Part model, mm, in its own coordinate system. Face numbers are marked on the shaded views. A direction names the side the tool comes from. Coordinates: 2 decimals unless noted, no trailing zeros. Loops run counter-clockwise (first coordinate to the right, second up) from the corner with the lowest first, then second, coordinate; pieces in that order, holes last. Notation, with made-up numbers: M 58,1.5 L 113,1.5 A16 cw 113,11.5 Z; hole C 48,51.5 d9. An arc over 180 degrees is marked long. Answer as a JSON object with one key per item and string values. Group by question number.
1. Mould opens along Z. For the marked faces 4, 5 and 6 say: released by +Z, released by -Z, zero draft, split by the parting line, or undercut.
2. 3-axis set-ups, long thin cutter, end or side, ignore diameter. For the marked faces 1, 2 and 3: which of +Z, -Z, +X, -X, +Y, -Y reach the whole face in a straight line?
3. Saw through at D-D on z = -27.5. Write the cut outline in (x, y).
4. Saw through at A-A on z = -37.5. Write the cut outline in (x, y), then the cut area to 3 significant figures.
5. Drill centre lines: L1, parallel to Z at x = -2.25, y = 8; L2, parallel to X at y = 1.6, z = 0; L3, parallel to Y at x = 3.25, z = -36. Where is each one in solid material? Low to high.
6. Drop flat-ended pins along their axis: pin 1 Ø1 at (x, z) = (0, -4.5) entering from +Y; pin 2 Ø2.5 at (x, z) = (0, -37.5) entering from +Y; pin 3 Ø9 at (x, z) = (9.5, -12) entering from -Y; pin 4 Ø3 at (x, z) = (6.5, -2) entering from -Y. Give the stop position or say it passes through.
7. Saw through at B-B on z = -18.75. Write the cut outline in (x, y).
8. Saw through at C-C on y = 39.5. Write the cut outline in (x, z), then the cut area to 3 significant figures.
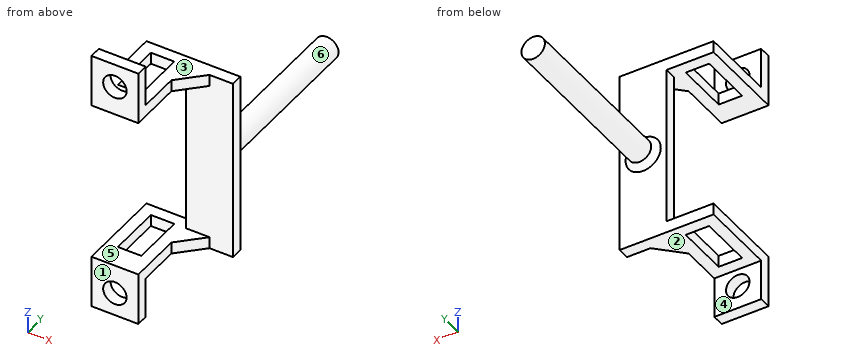
from build123d import *

# Parameters (mm, degrees)
SKETCH1_W             = 8
SKETCH1_H             = 8
SKETCH1_R             = 2
BOSS_EXTRUDE1_DEPTH   = 2
BOSS_EXTRUDE1_2_DEPTH = 2
SKETCH2_W             = 8
SKETCH2_H             = 2
BOSS_EXTRUDE2_DEPTH   = 15
BOSS_EXTRUDE3_REACH   = 43.512
SKETCH3_W             = 8
SKETCH3_H             = 2
CHAMFER1_SIZE         = 4
SKETCH4_W             = 4
SKETCH4_H             = 9
CUT_EXTRUDE1_DEPTH    = 44.026154836
SKETCH5_R             = 2
BOSS_EXTRUDE4_DEPTH   = 30
CHAMFER2_SIZE         = 1


with BuildPart() as part:
    # Sketch1 → Boss-Extrude1 (new body)
    with BuildSketch(Plane(origin=(0, 0, 0), x_dir=(1, 0, 0), z_dir=(0, 1, 0))):
        Rectangle(SKETCH1_W, SKETCH1_H)
        with Locations(Location((0, 0, 0), (0, 0, 270))):
            Circle(SKETCH1_R, mode=Mode.SUBTRACT)
    extrude(amount=BOSS_EXTRUDE1_DEPTH)



with BuildPart() as body_2:
    # Sketch1 → Boss-Extrude1 2 (new body)
    with BuildSketch(Plane(origin=(0, 0, 0), x_dir=(1, 0, 0), z_dir=(0, 1, 0))):
        with Locations((0, 37.5)):
            Rectangle(SKETCH1_W, SKETCH1_H)
        with Locations(Location((0, 37.5, 0), (0, 0, 270))):
            Circle(SKETCH1_R, mode=Mode.SUBTRACT)
    extrude(amount=BOSS_EXTRUDE1_2_DEPTH)


with BuildPart() as part_1:
    add(part.part)

    add(body_2.part)  # Boss-Extrude2 merges body 2
    # Sketch2 → Boss-Extrude2 (add)
    with BuildSketch(Plane.XZ):
        with Locations((0, -33.5)):
            Rectangle(SKETCH2_W, SKETCH2_H)
        with Locations((0, -4)):
            Rectangle(SKETCH2_W, SKETCH2_H)
    extrude(amount=-BOSS_EXTRUDE2_DEPTH)

    # Boss-Extrude3: up to this face of the body (flat: up to its plane)
    boss_extrude3_end = Plane(part_1.part.faces().sort_by_distance((0, 8.5, -3))[0])
    # Sketch3 → Boss-Extrude3 (add, up to the picked face)
    with BuildSketch(Plane.XY.offset(-34.5), mode=Mode.PRIVATE) as boss_extrude3_sk1:
        with Locations((8, 14)):
            Rectangle(SKETCH3_W, SKETCH3_H)
    boss_extrude3_tool1 = split(extrude(boss_extrude3_sk1.sketch, amount=BOSS_EXTRUDE3_REACH, mode=Mode.PRIVATE), bisect_by=boss_extrude3_end, keep=Keep.BOTH, mode=Mode.PRIVATE)
    add(boss_extrude3_tool1.solids().sort_by(Axis((8, 14, -34.5), (0, 0, 1)))[0])

    # Chamfer1
    chamfer1_edges = [part_1.edges().sort_by_distance(p)[0] for p in [
        (4, 13, -4),
        (4, 13, -33.5),
    ]]
    chamfer(chamfer1_edges, length=CHAMFER1_SIZE)

    # Sketch4 → Cut-Extrude1 (cut, through all)
    with BuildSketch(Plane.XY.offset(-3)):
        with Locations((0, 8.5)):
            Rectangle(SKETCH4_W, SKETCH4_H)
    extrude(amount=-CUT_EXTRUDE1_DEPTH, mode=Mode.SUBTRACT)

    # Sketch5 → Boss-Extrude4 (add)
    with BuildSketch(Plane(origin=(0, 15, 0), x_dir=(1, 0, 0), z_dir=(0, 1, 0))):
        with Locations(Location((8, 18.75, 0), (0, 0, 90))):
            Circle(SKETCH5_R)
    extrude(amount=BOSS_EXTRUDE4_DEPTH)

    # Chamfer2
    chamfer2_edges = [part_1.edges().sort_by_distance(p)[0] for p in [
        (8, 15, -16.75),
    ]]
    chamfer(chamfer2_edges, length=CHAMFER2_SIZE)


solid = part_1.part
Outcome:
{
 "1": {"face 4": "zero draft", "face 5": "undercut", "face 6": "split by the parting line"},
 "2": {"face 1": "+Z, -Z, +X, -X, -Y", "face 2": "-Z, +X, -X, +Y", "face 3": "+Z, +X, -X, +Y"},
 "3": {"outline": "M 4,13 L 12,13 L 12,15 L 4,15 Z"},
 "4": {"outline": "M -4,0 L -2,0 L -2,2 L -4,2 Z; M 2,0 L 4,0 L 4,2 L 2,2 Z", "area": "8.00 mm²"},
 "5": {"L1": "z = -34.5 to -32.5, -5 to -3", "L2": "x = -4 to -2, 2 to 4", "L3": "y = 0 to 2"},
 "6": {"pin 1": "stops at y = 15", "pin 2": "passes through", "pin 3": "stops at y = 13", "pin 4": "stops at y = 10.38"},
 "7": {"outline": "M 4,13 L 12,13 L 12,15 L 11,15 L 10,16 L 10,45 L 6,45 L 6,16 L 5,15 L 4,15 Z"},
 "8": {"outline": "C 8,-18.75 d4", "area": "12.6 mm²"}
}
